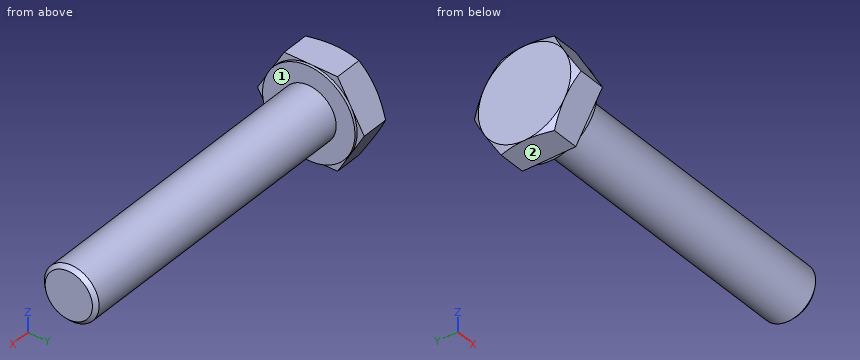
```python
from build123d import *

# Parameters (mm, degrees)
BASEHEAD_DEPTH = 10
SKETCH4_W      = 0.8
SKETCH4_H      = 12.088457268


# Read off the part's stored shape, not the designer's step: HeadChamfer
with BuildPart() as part:
    # Sketch1 → BaseHead (new body)
    with BuildSketch(Plane(origin=(0, 0, 0), x_dir=(0, 0, -1), z_dir=(1, 0, 0))):
        Polygon((13.5, 7.794228634), (13.5, -7.794228634), (0, -15.588457268), (-13.5, -7.794228634), (-13.5, 7.794228634), (0, 15.588457268), align=None)
    extrude(amount=BASEHEAD_DEPTH)

    # HeadChamfer outline → HeadChamfer (revolve, cut)
    with BuildSketch(Plane.YX):
        Polygon((15.58845727, 1.205771367), (13.499999851, -8.6e-08), (15.58845727, -8.6e-08), align=None)
    revolve(axis=Axis((0, 0, 0), (1, 0, 0)), mode=Mode.SUBTRACT)

    # HeadChamfer 2 outline → HeadChamfer 2 (revolve)
    with BuildSketch(Plane.YX):
        Polygon((8, 10), (8, 98.8985), (6.8985, 100), (0, 100), (0, 10), align=None)
    revolve(axis=Axis((0, 0, 0), (1, 0, 0)))

    # Sketch4 → BearingFace (revolve, cut)
    with BuildSketch(Plane.XY, mode=Mode.PRIVATE) as bearingface_sk:
        with Locations((9.6, 19.544228634)):
            Rectangle(SKETCH4_W, SKETCH4_H)
    revolve(bearingface_sk.sketch.rotate(Axis((0, 0, 0), (1, 0, 0)), 90), axis=Axis((0, 0, 0), (1, 0, 0)), mode=Mode.SUBTRACT)


solid = part.part
```
Build history of the part. All positions in model axes, mm. Face numbers are marked on the shaded views. A direction names the side the tool comes from. Round coordinates to 2 decimals unless told otherwise and drop trailing zeros. Write each loop counter-clockwise with the first axis right and the second up, starting at its lowest first coordinate (ties: lowest second). Pieces come first, ordered by that corner, then holes. Notation, with made-up numbers: (71.25, -21) -> (102.25, -21) arc R30 ccw to (102.25, 1) -> close; hole circle Ø11 at (41, -23). An arc over 180 degrees is marked (long way). Put each result on its own line as item: value.
Item 1: Flat gauge pins, fed straight in: P1, Ø1.2, axis at y = -14, z = -2.5, coming from the +X side; P2, Ø1.2, axis at y = 13, z = 1.5, coming from the +X side; P3, Ø8, axis at y = 9.5, z = 10.5, coming from the -X side; P4, Ø8, axis at x = 59, y = 0, coming from the -Z side. Where does each tip first touch, or does it go through?
Here are the results:
P1: stops at x = 9.2
P2: stops at x = 10
P3: stops at x = 0
P4: stops at z = -8
Item 2: Wall check: probe 1 along X at (y, z) = (9.5, -3.25); probe 2 along Z at (x, y) = (45, 0.5); probe 3 along Y at (x, z) = (65, -0.25). Give the ranges that are in metal, low to high. Write a range as from..to.
Here are the results:
probe 1: x = 0..10
probe 2: z = -7.98..7.98
probe 3: y = -8..8
Item 3: Tool access for the marked faces 1 and 2: list every direction of +Z, -Z, +X, -X, +Y, -Y with a clear straight run to the whole face (end or side of a thin tool).
Here are the results:
face 1: +X
face 2: -Z, +X, -X, +Y, -Y
Item 4: Slice it at A-A, the plane x = 71.5. Give the cut face in (y, z), plus the area to 3 significant figures.
Here are the results:
outline: circle Ø16 at (0, 0)
area: 201 mm^2
